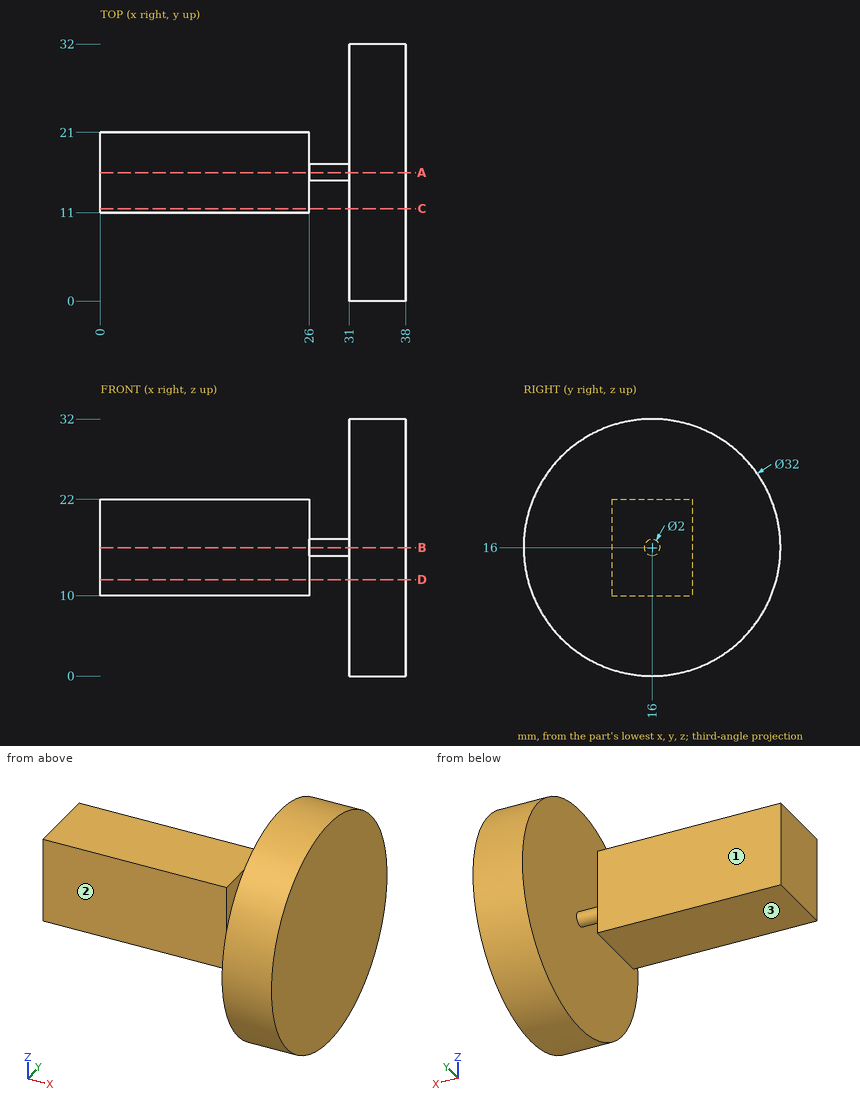
Answer from the drawing. Dimensions are ordinates in mm from the lowest x, y and z of the part. A direction names the side the tool comes from. Give positions to 0.01 mm unless a question says otherwise; leave off trailing zeros. Loops run counter-clockwise (first coordinate to the right, second up) from the corner with the lowest first, then second, coordinate; pieces in that order, holes last. Notation, with made-up numbers: (-37.75, 87) -> (-6.75, 87) arc R30 ccw to (-6.75, 112) -> close; hole circle Ø4 at (-4.5, 66). An arc over 180 degrees is marked (long way). Use a Markdown table: item, result.
Q1. Section D-D, the plane z = 12 is taken. Determine the outline of the cut face in (x, y), then the cut area to 3 significant figures.
Solved:
| item | result |
|---|---|
| outline | (0, 11) -> (26, 11) -> (26, 21) -> (0, 21) -> close; (31, 0.51) -> (38, 0.51) -> (38, 31.49) -> (31, 31.49) -> close |
| area | 477 mm^2 |
Q2. Section B-B, the plane z = 16 is taken. Determine the outline of the cut face in (x, y).
Solved:
| item | result |
|---|---|
| outline | (0, 11) -> (26, 11) -> (26, 15) -> (31, 15) -> (31, 0) -> (38, 0) -> (38, 32) -> (31, 32) -> (31, 17) -> (26, 17) -> (26, 21) -> (0, 21) -> close |
Q3. Section A-A, the plane y = 16 is taken. Determine the outline of the cut face in (x, z), then the cut area to 3 significant figures.
Solved:
| item | result |
|---|---|
| outline | (0, 10) -> (26, 10) -> (26, 15) -> (31, 15) -> (31, 0) -> (38, 0) -> (38, 32) -> (31, 32) -> (31, 17) -> (26, 17) -> (26, 22) -> (0, 22) -> close |
| area | 546 mm^2 |
Q4. Section C-C, the plane y = 11.5 is taken. Determine the outline of the cut face in (x, z).
Solved:
| item | result |
|---|---|
| outline | (0, 10) -> (26, 10) -> (26, 22) -> (0, 22) -> close; (31, 0.65) -> (38, 0.65) -> (38, 31.35) -> (31, 31.35) -> close |
Q5. Find the intervals of material crossed by line 1 along X through (y, z) = (26, 18); line 2 along Y through (x, z) = (5, 16); line 3 along Y through (x, z) = (31.5, 16), in increasing order.
Solved:
| item | result |
|---|---|
| line 1 | x = 31 to 38 |
| line 2 | y = 11 to 21 |
| line 3 | y = 0 to 32 |
Q6. A tool of negligible diameter and unlimited length cuts with its end or side. For the marked faces 1, 2 and 3, from which of +Z, -Z, +X, -X, +Y, -Y can it reach the whole face along a straight path? Write none if from no direction.
Solved:
| item | result |
|---|---|
| face 1 | +Z, -Z, -X, +Y |
| face 2 | +Z, -Z, -X, -Y |
| face 3 | -Z, -X, +Y, -Y |
Q7. Each of these flat-tipped pins is pushed along its axis until it touches: pin 1 (5 mm diameter, centred on x = 18, y = 14.5, fed in from -Z); pin 2 (1.5 mm diameter, centred on y = 3, z = 22, fed in from -X); pin 3 (3 mm diameter, centred on x = 30, z = 7.5, fed in from -Y). Where does it stop, or does it pass through?
Solved:
| item | result |
|---|---|
| pin 1 | stops at z = 10 |
| pin 2 | stops at x = 31 |
| pin 3 | stops at y = 1.8 |
